```python
from build123d import *

# Parameters (mm, degrees)
SKETCH1_R           = 5.085
BOSS_EXTRUDE1_DEPTH = 23.23
SKETCH2_R           = 5.085
SKETCH2_R_2         = 2
CUT_EXTRUDE1_DEPTH  = 1
SKETCH4_R           = 0.8
CUT_EXTRUDE2_DEPTH  = 0.5
SKETCH5_W           = 3.99879876
SKETCH5_H           = 10.17
SKETCH5_W_2         = 3.491908776
CUT_EXTRUDE3_DEPTH  = 12.47
CUT_EXTRUDE4_START  = -3.71
SKETCH6_R           = 5.085
SKETCH6_R_2         = 2.25
CUT_EXTRUDE4_DEPTH  = 3.71
SKETCH7_R           = 3.63
SKETCH7_R_2         = 3.57
CUT_EXTRUDE5_DEPTH  = 0.1
CUT_EXTRUDE6_START  = -0.68
SKETCH8_R           = 2.25
SKETCH8_R_2         = 0.715
CUT_EXTRUDE6_DEPTH  = 0.68
CUT_EXTRUDE7_START  = -3.03
CUT_EXTRUDE7_DEPTH  = 3.03
SKETCH10_R          = 0.455
BOSS_EXTRUDE2_DEPTH = 0.68
CUT_EXTRUDE8_START  = 0.01
SKETCH11_R          = 5.085
SKETCH11_R_2        = 5.035
CUT_EXTRUDE8_DEPTH  = 0.01
FILLET3_R           = 0.2
CUT_EXTRUDE9_DEPTH  = 0.01


with BuildPart() as part:
    # Sketch1 → Boss-Extrude1 (new body)
    with BuildSketch(Plane.XY):
        Circle(SKETCH1_R)
    extrude(amount=BOSS_EXTRUDE1_DEPTH)

    # Sketch2 → Cut-Extrude1 (cut)
    with BuildSketch(Plane(origin=(0, 0, 0), x_dir=(-1, 0, 0), z_dir=(0, 0, -1))):
        Circle(SKETCH2_R)
        Circle(SKETCH2_R_2, mode=Mode.SUBTRACT)
    extrude(amount=-CUT_EXTRUDE1_DEPTH, mode=Mode.SUBTRACT)

    # Sketch4 → Cut-Extrude2 (cut)
    with BuildSketch(Plane(origin=(0, 0, 0), x_dir=(-1, 0, 0), z_dir=(0, 0, -1))):
        Circle(SKETCH4_R)
    extrude(amount=-CUT_EXTRUDE2_DEPTH, mode=Mode.SUBTRACT)

    # Sketch5 → Cut-Extrude3 (cut)
    with BuildSketch(Plane(origin=(0, 0, 0), x_dir=(-1, 0, 0), z_dir=(0, 0, -1))):
        with Locations((6.04439938, 0)):
            Rectangle(SKETCH5_W, SKETCH5_H)
        with Locations((-5.790954388, 0)):
            Rectangle(SKETCH5_W_2, SKETCH5_H)
    extrude(amount=-CUT_EXTRUDE3_DEPTH, mode=Mode.SUBTRACT)

    # Sketch6 → Cut-Extrude4 (cut)
    with BuildSketch(Plane.XY.offset(23.23).offset(CUT_EXTRUDE4_START)):
        with Locations(Location((0, 0, 0), (0, 0, 142.7003226))):
            Circle(SKETCH6_R)
        Circle(SKETCH6_R_2, mode=Mode.SUBTRACT)
    extrude(amount=CUT_EXTRUDE4_DEPTH, mode=Mode.SUBTRACT)

    # Sketch7 → Cut-Extrude5 (cut)
    with BuildSketch(Plane.XY.offset(19.52)):
        Circle(SKETCH7_R)
        Circle(SKETCH7_R_2, mode=Mode.SUBTRACT)
    extrude(amount=-CUT_EXTRUDE5_DEPTH, mode=Mode.SUBTRACT)

    # Sketch8 → Cut-Extrude6 (cut)
    with BuildSketch(Plane.XY.offset(23.23).offset(CUT_EXTRUDE6_START)):
        Circle(SKETCH8_R)
        Circle(SKETCH8_R_2, mode=Mode.SUBTRACT)
    extrude(amount=CUT_EXTRUDE6_DEPTH, mode=Mode.SUBTRACT)

    # Sketch9 → Cut-Extrude7 (cut)
    with BuildSketch(Plane.XY.offset(22.55).offset(CUT_EXTRUDE7_START)):
        with BuildLine():
            ThreePointArc((-1.018056831, 1.101617125), (-0.75, 1.299038106), (-0.445, 1.43247164))
            Line((-0.445, 1.43247164), (-0.445, 2.205555486))
            ThreePointArc((-0.445, 2.205555486), (-1.125, 1.948557159), (-1.68756708, 1.488159047))
            Line((-1.68756708, 1.488159047), (-1.018056831, 1.101617125))
        make_face()
        with BuildLine():
            Line((0.445, 2.205555486), (0.445, 1.43247164))
            ThreePointArc((0.445, 1.43247164), (0.75, 1.299038106), (1.018056831, 1.101617125))
            Line((1.018056831, 1.101617125), (1.68756708, 1.488159047))
            ThreePointArc((1.68756708, 1.488159047), (1.125, 1.948557159), (0.445, 2.205555486))
        make_face()
        with BuildLine():
            Line((2.13256708, 0.717396438), (1.463056831, 0.330854515))
            ThreePointArc((1.463056831, 0.330854515), (1.490735598, 0.16645533), (1.5, 0))
            ThreePointArc((1.5, 0), (1.490735598, -0.16645533), (1.463056831, -0.330854515))
            Line((1.463056831, -0.330854515), (2.13256708, -0.717396438))
            ThreePointArc((2.13256708, -0.717396438), (2.220447695, -0.363472193), (2.25, 0))
            ThreePointArc((2.25, 0), (2.220447695, 0.363472193), (2.13256708, 0.717396438))
        make_face()
        with BuildLine():
            Line((1.68756708, -1.488159047), (1.018056831, -1.101617125))
            ThreePointArc((1.018056831, -1.101617125), (0.75, -1.299038106), (0.445, -1.43247164))
            Line((0.445, -1.43247164), (0.445, -2.205555486))
            ThreePointArc((0.445, -2.205555486), (1.125, -1.948557159), (1.68756708, -1.488159047))
        make_face()
        with BuildLine():
            ThreePointArc((-0.445, -1.43247164), (-0.75, -1.299038106), (-1.018056831, -1.101617125))
            Line((-1.018056831, -1.101617125), (-1.68756708, -1.488159047))
            ThreePointArc((-1.68756708, -1.488159047), (-1.125, -1.948557159), (-0.445, -2.205555486))
            Line((-0.445, -2.205555486), (-0.445, -1.43247164))
        make_face()
        with BuildLine():
            ThreePointArc((-1.463056831, -0.330854515), (-1.5, 0), (-1.463056831, 0.330854515))
            Line((-1.463056831, 0.330854515), (-2.13256708, 0.717396438))
            ThreePointArc((-2.13256708, 0.717396438), (-2.25, 0), (-2.13256708, -0.717396438))
            Line((-2.13256708, -0.717396438), (-1.463056831, -0.330854515))
        make_face()
    extrude(amount=CUT_EXTRUDE7_DEPTH, mode=Mode.SUBTRACT)

    # Sketch10 → Boss-Extrude2 (add)
    with BuildSketch(Plane(origin=(0, 0, 1), x_dir=(-1, 0, 0), z_dir=(0, 0, -1))):
        with Locations((2.5, -3.145160742)):
            Circle(SKETCH10_R)
    extrude(amount=BOSS_EXTRUDE2_DEPTH)

    # Sketch11 → Cut-Extrude8 (cut)
    with BuildSketch(Plane(origin=(0, 0, 12.47), x_dir=(-1, 0, 0), z_dir=(0, 0, -1)).offset(CUT_EXTRUDE8_START)):
        Circle(SKETCH11_R)
        Circle(SKETCH11_R_2, mode=Mode.SUBTRACT)
    extrude(amount=-CUT_EXTRUDE8_DEPTH, mode=Mode.SUBTRACT)

    # Fillet3
    # the kernel refuses this fillet: 0.2 mm, written as the material it takes off along each edge
    with BuildSketch(Plane(origin=(0, 0, 12.46), x_dir=(-0.8331991700608187, 0.5529730038708609, 0), z_dir=(-0.5529730038708609, -0.8331991700608187, 0))) as fillet3_piece_1:
        with BuildLine():
            CenterArc((4.885, 0.132287566), FILLET3_R, 318.590377891, 41.409622109)
            Line((5.035, 0), (5.085, 0))
            Line((5.085, 0), (5.085, 0.132287566))
        make_face()
    fillet3_piece_1_solid = revolve(axis=Axis((0, 0, 12.46), (0, 0, -1)), revolution_arc=112.857572989, mode=Mode.PRIVATE)
    with BuildSketch(Plane(origin=(0, 0, 12.46), x_dir=(0.8331991700608224, -0.5529730038708549, 0), z_dir=(0.5529730038708549, 0.8331991700608224, 0))) as fillet3_piece_2:
        with BuildLine():
            CenterArc((4.885, 0.132287566), FILLET3_R, 318.590377891, 41.409622109)
            Line((5.085, 0.132287566), (5.085, 0))
            Line((5.085, 0), (5.035, 0))
        make_face()
    fillet3_piece_2_solid = revolve(axis=Axis((0, 0, 12.46), (0, 0, -1)), revolution_arc=112.857572989, mode=Mode.PRIVATE)
    with BuildSketch(Plane(origin=(-4.045, 3.08142824, 12.46), x_dir=(0.6114168469415571, 0.7913086877294123, 0), z_dir=(0, 0, -1))) as fillet3_piece_3:
        with BuildLine():
            CenterArc((0.068270891, 0.199995311), FILLET3_R, 232.307979121, 38.084364359)
            Line((-0.054012478, 0.041733573), (0, 0))
            ThreePointArc((0, 0), (0.034820209, -0.000119219), (0.069640417, 0))
        make_face()
    fillet3_piece_3_solid = extrude(amount=11.634101044, mode=Mode.PRIVATE)
    with BuildSketch(Plane(origin=(-4.045, -3.08142824, 12.46), x_dir=(0.6114168469415588, -0.7913086877294109, 0), z_dir=(0, 0, -1)), Plane(origin=(4.045, 3.08142824, 12.46), x_dir=(-0.6114168469415571, 0.7913086877294123, 0), z_dir=(0, 0, -1))) as fillet3_piece_4:
        with BuildLine():
            CenterArc((0.068270891, -0.199995311), FILLET3_R, 89.60765652, 38.084364359)
            Line((-0.054012478, -0.041733573), (0, 0))
            ThreePointArc((0, 0), (0.034820209, 0.000119219), (0.069640417, 0))
        make_face()
    fillet3_piece_4_solid = extrude(amount=11.634101044, mode=Mode.PRIVATE)
    with BuildSketch(Plane(origin=(4.045, -3.08142824, 12.46), x_dir=(0, 1, 0), z_dir=(0, 0, -1))) as fillet3_piece_5:
        with BuildLine():
            CenterArc((0.068257153, -0.2), FILLET3_R, 90, 38.084364359)
            ThreePointArc((-0.055107067, -0.042579324), (-0.027626426, -0.021195323), (0, 0))
            Line((0, 0), (0.068257153, 0))
        make_face()
    fillet3_piece_5_solid = extrude(amount=11.634101044, mode=Mode.PRIVATE)
    add([fillet3_piece_1_solid, fillet3_piece_2_solid, fillet3_piece_3_solid, fillet3_piece_4_solid, fillet3_piece_5_solid], mode=Mode.SUBTRACT)

    # Sketch15 → Cut-Extrude9 (cut)
    with BuildSketch(Plane(origin=(0, 0, 1.5), x_dir=(-1, 0, 0), z_dir=(0, 0, -1))):
        with BuildLine():
            Line((4.045, -3.013171087), (4.045, 3.013171087))
            ThreePointArc((4.045, 3.013171087), (4.034055726, 3.078423922), (4.002420676, 3.136535308))
            ThreePointArc((4.002420676, 3.136535308), (0, 5.085), (-4.002420676, 3.136535308))
            ThreePointArc((-4.002420676, 3.136535308), (-4.034055726, 3.078423922), (-4.045, 3.013171087))
            Line((-4.045, 3.013171087), (-4.045, -3.013171087))
            ThreePointArc((-4.045, -3.013171087), (-4.034055726, -3.078423922), (-4.002420676, -3.136535308))
            ThreePointArc((-4.002420676, -3.136535308), (0, -5.085), (4.002420676, -3.136535308))
            ThreePointArc((4.002420676, -3.136535308), (4.034055726, -3.078423922), (4.045, -3.013171087))
        make_face()
        with BuildLine():
            Line((-3.945, 3.120556841), (-3.945, -3.120556841))
            ThreePointArc((-3.945, -3.120556841), (0, -5.03), (3.945, -3.120556841))
            Line((3.945, -3.120556841), (3.945, 3.120556841))
            ThreePointArc((3.945, 3.120556841), (-0.000264914, 5.029999993), (-3.945, 3.120556841))
        make_face(mode=Mode.SUBTRACT)
    extrude(amount=-CUT_EXTRUDE9_DEPTH, mode=Mode.SUBTRACT)


solid = part.part
```
Work out the finished part from the listing and answer in its coordinate system (mm). A direction names the side the tool comes from. Coordinates: 2 decimals unless noted, no trailing zeros. Loops run counter-clockwise (first coordinate to the right, second up) from the corner with the lowest first, then second, coordinate; pieces in that order, holes last. Notation, with made-up numbers: M 27,22.25 L 66,22.25 A25 ccw 66,59.25 Z; hole C 8,11 d10. An arc over 180 degrees is marked long. Use CSV: the item, a comma, the result in double quotes. Start each with the question number.
(1) Consider line 1 (Y direction, x = 0, z = 0.35); line 2 (Z direction, x = -4.5, y = -1.5); line 3 (Y direction, x = 0.25, z = 12.5). Determine where each line is inside the solid, lowest interval first.
(2) Find section B-B, the plane z = 22. Give the vertices of the cut face in (x, y) (3 decimals).
(3) Given pin 1 Ø1 at (x, y) = (0, 0) entering from -Z; pin 2 Ø1.5 at (y, z) = (-2, 6) entering from -X (3 decimals); pin 3 Ø2 at (y, z) = (1.5, 12.5) entering from -X, each flat-ended and moving along its own axis, determine where each tip first touches the part or whether it passes through.
(4) For a pull along Y with two mould halves and no side action, classify faces 1 (the face through (0, 0, 23.23)), 2 (the face through (0, 0, 0.5)), 3 (the face through (0.065, 5.085, 1.246)) as +Y half, -Y half, draft (parallel to the pull), parting line (faces both ways), or undercut.
(5) For faces 4 (the face through (2, 1, 1)), 5 (the face through (4.045, 0, 7)), 6 (the face through (-0.01, -2.25, 21.01)), 7 (the face through (-4.045, 0, 7)), 8 (the face through (0, 4, 19.52)), determine the directions among +Z, -Z, +X, -X, +Y, -Y from which every point of the face is accessible in a straight line to the end or side of a thin tool.
(6) Find section A-A, the plane z = 10.5. Give the vertices of the cut face in (x, y) (3 decimals).
Recorded:
1,line 1,"y = -2 to -0.8, 0.8 to 2"
1,line 2,"z = 12.47 to 19.52"
1,line 3,"y = -5.08 to 5.08"
2,outline,"M -2.133,-0.717 A2.25 ccw -1.688,-1.488 L -1.018,-1.102 A1.5 ccw -0.445,-1.432 L -0.445,-2.206 A2.25 ccw 0.445,-2.206 L 0.445,-1.432 A1.5 ccw 1.018,-1.102 L 1.688,-1.488 A2.25 ccw 2.133,-0.717 L 1.463,-0.331 A1.5 ccw 1.463,0.331 L 2.133,0.717 A2.25 ccw 1.688,1.488 L 1.018,1.102 A1.5 ccw 0.445,1.432 L 0.445,2.206 A2.25 ccw -0.445,2.206 L -0.445,1.432 A1.5 ccw -1.018,1.102 L -1.688,1.488 A2.25 ccw -2.133,0.717 L -1.463,0.331 A1.5 ccw -1.463,-0.331 Z"
3,pin 1,"stops at z = 0.5"
3,pin 2,"stops at x = -4.045"
3,pin 3,"stops at x = -5.06"
4,face 1,"draft"
4,face 2,"undercut"
4,face 3,"+Y half"
5,face 4,"-Z"
5,face 5,"-Z, +X, +Y, -Y"
5,face 6,"+Z, -Y"
5,face 7,"-Z, -X, +Y, -Y"
5,face 8,"+Z"
6,outline,"M -4.045,-3.013 A0.2 ccw -4.002,-3.137 A5.085 ccw 4.002,-3.137 A0.2 ccw 4.045,-3.013 L 4.045,3.013 A0.2 ccw 4.002,3.137 A5.085 ccw -4.002,3.137 A0.2 ccw -4.045,3.013 Z"
